Could you check a few things on this model? Use its own coordinates, in mm. Face numbers are marked on the shaded views. A direction names the side the tool comes from. Round coordinates to 2 decimals unless told otherwise and drop trailing zeros. Loops run counter-clockwise (first coordinate to the right, second up) from the corner with the lowest first, then second, coordinate; pieces in that order, holes last. Notation, with made-up numbers: (64.5, -15) -> (87.5, -15) arc R14 cw to (87.5, -4) -> close; hole circle Ø6 at (-22, 16). An arc over 180 degrees is marked (long way). One line per item, written item: value.
```python
from build123d import *

# Parameters (mm, degrees)
SKETCH1_W           = 20
SKETCH1_H           = 10
BOSS_EXTRUDE1_DEPTH = 5
BOSS_EXTRUDE2_DEPTH = 20
CUT_EXTRUDE1_DEPTH  = 4.09576
FILLET1_R           = 0.5


with BuildPart() as part:
    # Sketch1 → Boss-Extrude1 (new body)
    with BuildSketch(Plane.XY):
        with Locations((-83, 16.5)):
            Rectangle(SKETCH1_W, SKETCH1_H)
    extrude(amount=BOSS_EXTRUDE1_DEPTH)

    # Sketch2 → Boss-Extrude2 (add)
    with BuildSketch(Plane.ZY.offset(93)):
        Polygon((5, 16.5), (1.498962309, 11.5), (6.498962309, 11.5), (32.208054955, 48.216389418), (32.208054955, 55.357129452), (8.501037691, 21.5), (5, 21.5), align=None)
    extrude(amount=-BOSS_EXTRUDE2_DEPTH)

    # Sketch3 → Cut-Extrude1 (cut)
    with BuildSketch(Plane(origin=(0, 3.079102266, -4.397413763), x_dir=(-1, 0, 0), z_dir=(0, 0.573576436, -0.819152044))):
        Polygon((90.5, 29.170685305), (90.5, 36.425657649), (86.606804382, 33.925761075), align=None)
        Polygon((76.580636571, 27.487763856), (89.293048323, 27.487763856), (84.912643674, 32.837907557), align=None)
        Polygon((79.020661139, 31.431370249), (75.5, 42.221469006), (75.5, 29.170685305), align=None)
        Polygon((83.682826439, 48.850072065), (75.5, 50.589500561), (75.5, 48.669091242), (77.437703633, 42.730430083), align=None)
        Polygon((77.812370658, 52.142645531), (81.816362113, 58.81968714), (75.5, 58.81968714), (75.5, 52.634187597), align=None)
        Polygon((90.5, 55.53027081), (90.5, 58.81968714), (84.148398738, 58.81968714), (83.395113947, 57.563512158), (88.334689519, 53.40846707), align=None)
        Polygon((86.899562452, 52.002175453), (85.397480311, 50.530274064), (79.880748536, 51.702969161), (82.353375162, 55.826312344), align=None)
        Polygon((90.5, 38.802476843), (90.5, 52.730114749), (88.38308654, 50.655735608), (88.38308654, 37.443165566), align=None)
        Polygon((86.38308654, 36.158926695), (80.76001209, 32.548241301), (78.130006045, 40.608666271), (86.38308654, 48.69592083), align=None)
    extrude(amount=-CUT_EXTRUDE1_DEPTH, mode=Mode.SUBTRACT)

    # Fillet1
    fillet1_edges = [part.edges().sort_by_distance(p)[0] for p in [
        (-88.38308654, 39.162299764, 20.868313128),
        (-90.5, 40.568657026, 21.853055085),
        (-89.44154327, 34.307489189, 17.468938167),
        (-89.44154327, 45.423467601, 25.252430045),
        (-85.864901733, 48.530564087, 27.428042427),
        (-90.5, 49.914103175, 28.396806926),
        (-87.324199369, 51.26136923, 29.340172774),
        (-89.41734476, 47.697797184, 26.844932764),
        (-83.771756342, 50.746870078, 28.979916589),
        (-84.626468807, 47.243065371, 26.526526121),
        (-81.117061849, 47.120517648, 26.440717281),
        (-82.639114423, 44.951387357, 24.9218759),
        (-86.148521381, 45.07393508, 25.007684739),
        (-88.553402191, 31.893356499, 15.778544259),
        (-88.553402191, 28.921893785, 13.697903667),
        (-90.5, 29.94579148, 14.414844551),
        (-83, 21.5, 8.501037691),
        (-83, 55.357129452, 32.208054955),
        (-83, 11.5, 6.498962309),
        (-93, 29.858194709, 19.353508632),
        (-93, 51.786759435, 32.208054955),
        (-93, 38.428564726, 20.354546323),
        (-73, 38.428564726, 20.354546323),
        (-73, 51.786759435, 32.208054955),
        (-73, 29.858194709, 19.353508632),
        (-83, 11.5, 0),
        (-93, 16.5, 0),
        (-73, 16.5, 0),
        (-80.560265036, 40.588280041, 21.866795268),
        (-76.468851816, 40.514154635, 21.814892099),
        (-79.59141322, 43.807166866, 24.120684086),
        (-75.5, 43.73304146, 24.068780918),
        (-73, 11.5, 3.249481154),
        (-93, 11.5, 3.249481154),
        (-76.656185329, 45.993180791, 25.651347516),
        (-79.814366386, 48.526613089, 27.425275908),
        (-93, 21.5, 4.250518846),
        (-78.658181056, 51.26136923, 29.340172774),
        (-75.5, 48.727936933, 27.566244381),
        (-73, 21.5, 4.250518846),
        (-87.102845999, 27.787050796, 12.903278052),
        (-80.746640123, 27.787050796, 12.903278052),
        (-82.936842447, 25.595760221, 11.368919873),
        (-77.26033057, 27.900251113, 12.982541767),
        (-77.26033057, 33.245539188, 16.725352771),
        (-75.5, 32.319616841, 16.077014963),
        (-86.38308654, 37.833613175, 19.937956762),
        (-82.256546293, 39.65611981, 21.214089647),
        (-79.445009068, 33.042417461, 16.583125407),
        (-83.571549315, 31.219910826, 15.306992522),
    ]]
    fillet(fillet1_edges, radius=FILLET1_R)


solid = part.part
```
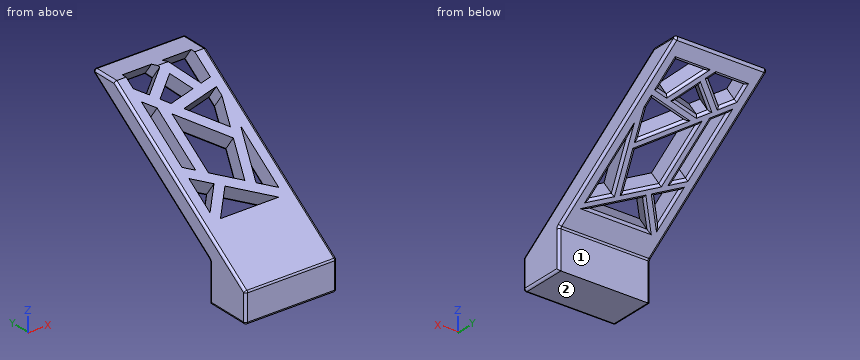
(1) Imagine slicing it at A-A on x = -91.5. Write out the boundary of the cut face in (y, z).
Results below:
outline: (11.5, 0.5) arc R0.5 ccw to (12, 0) -> (21.5, 0) -> (21.5, 8.24) arc R0.5 cw to (21.71, 8.65) -> (54.06, 31.3) arc R0.5 ccw to (53.77, 32.21) -> (48.22, 32.21) -> (11.71, 6.65) arc R0.5 ccw to (11.5, 6.24) -> close
(2) For pin 1 Ø2.5 at (x, z) = (-84.5, 2.5) entering from +Y; pin 2 Ø2 at (x, z) = (-82.5, 24.5) entering from -Y; pin 3 Ø10 at (x, y) = (-81.5, 49.5) entering from -Z, each with a flat end and sliding along its axis, tell me the tip position at first contact or that it passes through.
Results below:
pin 1: stops at y = 21.5
pin 2: stops at y = 36.74
pin 3: stops at z = 24.61
(3) Please list where these lines run through material, in increasing order: L1, parallel to X at y = 47.5, z = 27.5; L2, parallel to X at y = 46.5, z = 28.5; L3, parallel to Y at x = -89.25, z = 5.
Results below:
L1: x = -93 to -89.64, -86.82 to -83.71, -81.67 to -79.34, -75.5 to -73
L2: x = -93 to -89.38, -87.11 to -84, -81.52 to -79.19, -75.5 to -73
L3: y = 11.5 to 21.5
(4) On a 3-axis mill with a long thin cutter (end or side, diameter ignored), from which of +Z, -Z, +X, -X, +Y, -Y can I reach the whole of each face in a straight line? I mean the marked faces 1 and 2. Say none if no direction works.
Results below:
face 1: -Z, +X, -X, +Y
face 2: -Z, +X, -X, +Y, -Y
